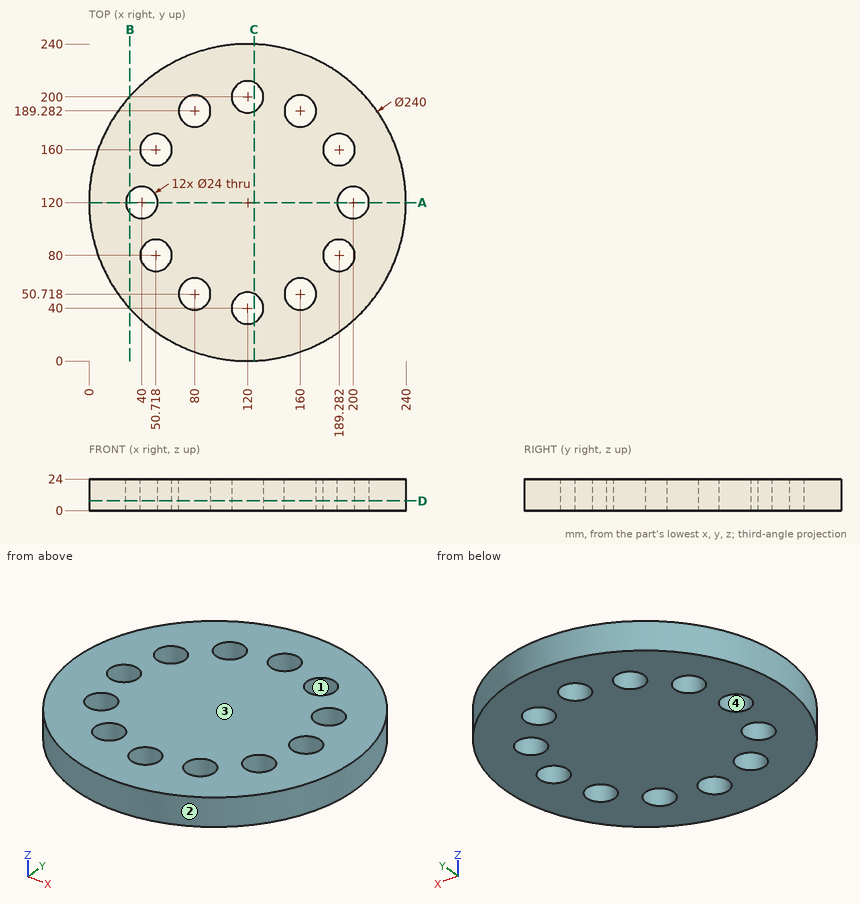
Input: dimensioned drawing with shaded views. Units: mm. Origin: part minimum x, y, z. Coordinates: 2 decimals unless noted, no trailing zeros. Loops run counter-clockwise (first coordinate to the right, second up) from the corner with the lowest first, then second, coordinate; pieces in that order, holes last. Notation, with made-up numbers: M 18,44.5 L 58,44.5 A8 ccw 58,59.5 Z; hole C 40,71.25 d9. An arc over 180 degrees is marked long. One line per item, written item: value.
(1) Section B-B (x = 31). Output: boundary loops of the cut face in (y, z).
Filled in:
outline: M 39.51,0 L 112.06,0 L 112.06,24 L 39.51,24 Z; M 127.94,0 L 200.49,0 L 200.49,24 L 127.94,24 Z
(2) Pin query (flat end, axial travel): pin 1 (21.5 mm diameter, centred on x = 80, y = 189.28, fed in from -Z); pin 2 (8 mm diameter, centred on x = 64, z = 8.5, fed in from -Y); pin 3 (3 mm diameter, centred on x = 95, z = 12, fed in from +Y); pin 4 (1 mm diameter, centred on x = 173.5, z = 5, fed in from -Y). Return the tip coordinate at first contact, or that it passes through.
Filled in:
pin 1: through
pin 2: y = 11.85
pin 3: y = 237.68
pin 4: y = 12.34
(3) Section C-C (x = 125). Output: boundary loops of the cut face in (y, z), and give its area (3 significant figures).
Filled in:
outline: M 0.1,0 L 29.09,0 L 29.09,24 L 0.1,24 Z; M 50.91,0 L 189.09,0 L 189.09,24 L 50.91,24 Z; M 210.91,0 L 239.9,0 L 239.9,24 L 210.91,24 Z
area: 4,710 mm^2
(4) Section A-A (y = 120). Output: boundary loops of the cut face in (x, z), and give its area (3 significant figures).
Filled in:
outline: M 0,0 L 28,0 L 28,24 L 0,24 Z; M 52,0 L 188,0 L 188,24 L 52,24 Z; M 212,0 L 240,0 L 240,24 L 212,24 Z
area: 4,610 mm^2
(5) Pull-direction query (X, two-part tool) for the marked faces 1, 2, 3 and 4; classes: +X half, -X half, draft (parallel to the pull), parting line (faces both ways), or undercut.
Filled in:
face 1: undercut
face 2: parting line
face 3: draft
face 4: undercut
(6) Line query: line 1 along Y through (x, z) = (120, 11.5); line 2 along Y through (x, z) = (179.5, 2.75); line 3 along Y through (x, z) = (47, 13.5). Output: solid intervals per line, ascending. Write a range as from..to.
Filled in:
line 1: 0..28, 52..188, 212..240
line 2: 15.79..73.05, 86.95..153.05, 166.95..224.21
line 3: 24.76..68.59, 91.41..110.25, 129.75..148.59, 171.41..215.24
(7) Section D-D (z = 7.5). Give the number of separate pieces and of enclosed holes in the cut face, and give its area (3 significant figures).
Filled in:
separate pieces: 1
enclosed holes: 12
area: 39,800 mm^2
